```python
from build123d import *

# Parameters (mm, degrees)
F1_DEPTH       = 10
F2_D           = 4.5
F2_CSINK_D     = 8.96
F2_CSINK_ANGLE = 90


with BuildPart() as f1:
    # F0 (on Front) → F1 (new body)
    with BuildSketch(Plane.XZ):
        Polygon((5, -11), (5, 40), (-5, 40), (-5, -11), (-5, -40), (5, -40), (5, -15), align=None)
        with BuildLine():
            ThreePointArc((10, -15), (8.461249695, -11.7984378813), (5, -11))
            Line((5, -11), (5, -15))
            Line((5, -15), (5, -40))
            Line((5, -40), (10, -40))
            Line((10, -40), (10, -15))
        make_face()
        with BuildLine():
            Line((-5, -40), (-5, -11))
            ThreePointArc((-5, -11), (-8.461249695, -11.7984378813), (-10, -15))
            Line((-10, -15), (-10, -40))
            Line((-10, -40), (-5, -40))
        make_face()
    extrude(amount=F1_DEPTH)

    # F2 (through all)
    with Locations(Plane(origin=(0, 0, 0), x_dir=(1, 0, 0), z_dir=(0, 1, 0))):
        with Locations((0, -14.3716754392), (0, 25.9504150599)):
            CounterSinkHole(F2_D / 2, F2_CSINK_D / 2, counter_sink_angle=F2_CSINK_ANGLE)


solid = f1.part
```
Model file for the job. Use its own axes, mm. Give positions to 0.01 mm unless a question says otherwise; leave off trailing zeros. Write each loop counter-clockwise with the first axis right and the second up, starting at its lowest first coordinate (ties: lowest second). Pieces come first, ordered by that corner, then holes. Notation, with made-up numbers: M 7.25,-32 L 38.25,-32 A29 cw 38.25,-8 Z; hole C 68.5,39 d8. An arc over 180 degrees is marked long. Use a Markdown table: item, result.
1) Drill centre lines: line 1 (Z direction, x = 0, y = -7); line 2 (Z direction, x = 1, y = -7); line 3 (X direction, y = -8, z = -26). Where is each one in solid material? Low to high. Write a range as from..to.
Responses:
| item | result |
|---|---|
| line 1 | z = -40..-28.2, -23.7..12.12, 16.62..40 |
| line 2 | z = -40..-27.97, -23.93..12.36, 16.39..40 |
| line 3 | x = -10..-2.25, 2.25..10 |
2) Pull direction Z, two halves, no side cores. Call faces 1 (the conical face through (0.31, -2.12, 12.03)), 2 (the flat face through (0, 0, -8)), 3 (the flat face through (0, -5, -40)): +Z half, -Z half, draft (parallel to the pull), parting line (faces both ways), or undercut.
Responses:
| item | result |
|---|---|
| face 1 | undercut |
| face 2 | draft |
| face 3 | -Z half |
3) Cut at D-D (x = -7.25). List the corners of the cut face in (y, z), and give its area (3 significant figures).
Responses:
| item | result |
|---|---|
| outline | M -10,-40 L 0,-40 L 0,-11.13 L -10,-11.13 Z |
| area | 289 mm2 |
4) Pin check, flat tip, straight feed: pin 1 (3.5 mm diameter, centred on x = 0, z = -25.95, fed in from -Y). Stop position of the tip, or through.
Responses:
| item | result |
|---|---|
| pin 1 | passes through |
5) Cut at A-A (x = 0). List the corners of the cut face in (y, z), and give its area (3 significant figures).
Responses:
| item | result |
|---|---|
| outline | M -10,-40 L 0,-40 L 0,-30.43 L -2.23,-28.2 L -10,-28.2 Z; M -10,-23.7 L -2.23,-23.7 L 0,-21.47 L 0,9.89 L -2.23,12.12 L -10,12.12 Z; M -10,16.62 L -2.23,16.62 L 0,18.85 L 0,40 L -10,40 Z |
| area | 700 mm2 |
6) Cut at C-C (z = 28). List the corners of the cut face in (x, y).
Responses:
| item | result |
|---|---|
| outline | M -5,-10 L 5,-10 L 5,0 L -5,0 Z |
7) Cut at B-B (y = -5.75). List the corners of the cut face in (x, z), and give its area (3 significant figures).
Responses:
| item | result |
|---|---|
| outline | M -10,-40 L 10,-40 L 10,-15 A4.1 ccw 5,-11 L 5,40 L -5,40 L -5,-11 A4.1 ccw -10,-15 Z; hole C 0,-25.95 d4.5; hole C 0,14.37 d4.5 |
| area | 1,050 mm2 |
